```python
from build123d import *

# Parameters (mm, degrees)
BOSS_EXTRUDE1_DEPTH          = 4.7625
F_3_8_0_375_DIAMETER_HOLE1_D = 9.525
F_3_4_0_75_DIAMETER_HOLE1_D  = 19.05
F_6_CLEARANCE_HOLE1_D        = 4.3053
FILLET1_R                    = 1.5875


with BuildPart() as part:
    # Sketch1 → Boss-Extrude1 (new body)
    with BuildSketch(Plane.XY):
        with BuildLine():
            Line((85.725, 56.35625), (85.725, 13.97))
            Line((85.725, 13.97), (66.675, 13.97))
            Line((66.675, 13.97), (66.675, 56.35625))
            Line((66.675, 56.35625), (11.2395, 56.35625))
            Line((11.2395, 56.35625), (11.2395, 42.8625))
            ThreePointArc((11.2395, 42.8625), (9.379628061, 38.372371939), (4.8895, 36.5125))
            Line((4.8895, 36.5125), (0.79375, 36.5125))
            Line((0.79375, 36.5125), (0.79375, 20.6375))
            Line((0.79375, 20.6375), (4.8895, 20.6375))
            ThreePointArc((4.8895, 20.6375), (9.379628061, 18.777628061), (11.2395, 14.2875))
            Line((11.2395, 14.2875), (11.2395, 0.79375))
            Line((11.2395, 0.79375), (134.8105, 0.79375))
            Line((134.8105, 0.79375), (134.8105, 14.2875))
            ThreePointArc((134.8105, 14.2875), (136.670371939, 18.777628061), (141.1605, 20.6375))
            Line((141.1605, 20.6375), (145.25625, 20.6375))
            Line((145.25625, 20.6375), (145.25625, 36.5125))
            Line((145.25625, 36.5125), (141.1605, 36.5125))
            ThreePointArc((141.1605, 36.5125), (136.670371939, 38.372371939), (134.8105, 42.8625))
            Line((134.8105, 42.8625), (134.8105, 56.35625))
            Line((134.8105, 56.35625), (85.725, 56.35625))
        make_face()
    extrude(amount=BOSS_EXTRUDE1_DEPTH)

    # 3/8 (0.375) Diameter Hole1 (through all)
    with Locations(Plane.XY.offset(4.7625)):
        with Locations((31.75, 24.13)):
            Hole(F_3_8_0_375_DIAMETER_HOLE1_D / 2)

    # 3/4 (0.75) Diameter Hole1 (through all)
    with Locations(Plane.XY.offset(4.7625)):
        with Locations((76.2, 28.575), (120.65, 28.575)):
            Hole(F_3_4_0_75_DIAMETER_HOLE1_D / 2)

    # #6 Clearance Hole1 (through all)
    with Locations(Plane.XY.offset(4.7625)):
        with Locations((19.05, 9.398), (19.05, 47.752), (127, 47.752), (127, 9.398)):
            Hole(F_6_CLEARANCE_HOLE1_D / 2)

    # Fillet1
    fillet1_edges = [part.edges().sort_by_distance(p)[0] for p in [
        (134.8105, 56.35625, 2.38125),
        (145.25625, 36.5125, 2.38125),
        (145.25625, 20.6375, 2.38125),
        (134.8105, 0.79375, 2.38125),
        (11.2395, 0.79375, 2.38125),
        (0.79375, 20.6375, 2.38125),
        (0.79375, 36.5125, 2.38125),
        (11.2395, 56.35625, 2.38125),
        (66.675, 13.97, 2.38125),
        (85.725, 13.97, 2.38125),
    ]]
    fillet(fillet1_edges, radius=FILLET1_R)


solid = part.part
```
Geometry check sheet. Reference: the model listing, model coordinates, mm. A direction names the side the tool comes from. Give positions to 0.01 mm unless a question says otherwise; leave off trailing zeros. Order: outer loops, then holes, each group sorted by start corner. A loop starts at its lowest first (then second) coordinate and runs counter-clockwise, first axis right, second up. Notation, with made-up numbers: (32, 31) - (87, 31) arc R10 cw to (87, 40) - close; hole circle Ø3 at (39.5, 60.25). An arc over 180 degrees is marked (long way). Answer in a Markdown table with one row per item. Add a question column.
Q1. Material ranges on probe 1 along Y at (x, z) = (19.05, 2.95); probe 2 along X at (y, z) = (29, 1.4) (3 decimals); probe 3 along X at (y, z) = (46, 2.3) (1 decimal), recorded low to high. Write a range as from..to.
Q2. Cross-section at B-B, the plane y = 24.13. Enter the section's corners in (x, z) (1 decimal).
Q3. Cross-section at C-C, the plane y = 17. Enter the section's corners in (x, z) (1 decimal), then the cut area to 3 significant figures.
Q4. Cross-section at A-A, the plane x = 31.75. Enter the section's corners in (y, z), then the cut area to 3 significant figures.
Q5. Mould release check, pull along X, two halves, no side actions. Record for faces 4 (the flat face through (56, 29, 4.762)), 5 (the cylindrical face through (136.72, 38.323, 2.348)), 6 (the flat face through (85.725, 36, 2)), 7 (the cylindrical face through (21.2, 9.5, 2.3)): pulls with the +X half, pulls with the -X half, needs draft (parallel to the pull), parting line crosses it, or undercut.
Q6. Cross-section at D-D, the plane x = 127. Enter the section's corners in (y, z).
Q7. Tool access check on faces 1 (the flat face through (4, 36.512, 2)), 2 (the flat face through (142, 20.638, 2)), 3 (the flat face through (11.24, 8, 2)). Record the directions out of +Z, -Z, +X, -X, +Y, -Y that give a thin tool (end or side, any length) a straight path to the whole face; none if there is none.
Q8. Gauge pin test, flat ends, axial feed: pin 1 (8.5 mm diameter, centred on x = 31.75, y = 24.13, fed in from -Z); pin 2 (0.8 mm diameter, centred on x = 142, z = 2, fed in from +Y); pin 3 (2.5 mm diameter, centred on x = 76, z = 1.5, fed in from +Y); pin 4 (1.4 mm diameter, centred on y = 48, z = 1.5, fed in from -X). Record the tip position at first contact, or that the pin passes through.
Check values:
| question | item | result |
|---|---|---|
| 1 | probe 1 | y = 0.79..7.25, 11.55..45.6, 49.9..56.36 |
| 1 | probe 2 | x = 0.794..66.675, 85.725..111.134, 130.166..145.256 |
| 1 | probe 3 | x = 11.2..17.8, 20.3..66.7, 85.7..125.7, 128.3..134.8 |
| 2 | outline | (0.8, 0) - (27, 0) - (27, 4.8) - (0.8, 4.8) - close; (36.5, 0) - (66.7, 0) - (66.7, 4.8) - (36.5, 4.8) - close; (85.7, 0) - (112.2, 0) - (112.2, 4.8) - (85.7, 4.8) - close; (129.1, 0) - (145.3, 0) - (145.3, 4.8) - (129.1, 4.8) - close |
| 3 | outline | (10.6, 0) - (66.7, 0) - (66.7, 4.8) - (10.6, 4.8) - close; (85.7, 0) - (135.4, 0) - (135.4, 4.8) - (85.7, 4.8) - close |
| 3 | area | 504 mm^2 |
| 4 | outline | (0.79, 0) - (19.37, 0) - (19.37, 4.76) - (0.79, 4.76) - close; (28.89, 0) - (56.36, 0) - (56.36, 4.76) - (28.89, 4.76) - close |
| 4 | area | 219 mm^2 |
| 5 | face 4 | needs draft |
| 5 | face 5 | pulls with the +X half |
| 5 | face 6 | undercut |
| 5 | face 7 | undercut |
| 6 | outline | (0.79, 0) - (7.25, 0) - (7.25, 4.76) - (0.79, 4.76) - close; (11.55, 0) - (21.48, 0) - (21.48, 4.76) - (11.55, 4.76) - close; (35.67, 0) - (45.6, 0) - (45.6, 4.76) - (35.67, 4.76) - close; (49.9, 0) - (56.36, 0) - (56.36, 4.76) - (49.9, 4.76) - close |
| 7 | face 1 | +Z, -Z, -X, +Y |
| 7 | face 2 | +Z, -Z, +X, -Y |
| 7 | face 3 | +Z, -Z, -X, -Y |
| 8 | pin 1 | passes through |
| 8 | pin 2 | stops at y = 36.51 |
| 8 | pin 3 | stops at y = 13.97 |
| 8 | pin 4 | stops at x = 11.24 |
